Verification items for the finished model (mm, model axes). Face numbers are marked on the shaded views. Coordinates: 2 decimals unless noted, no trailing zeros. Loops run counter-clockwise (first coordinate to the right, second up) from the corner with the lowest first, then second, coordinate; pieces in that order, holes last. Notation, with made-up numbers: (9.5, 70) -> (53.5, 70) arc R12 ccw to (53.5, 89) -> close; hole circle Ø8 at (16, 40). An arc over 180 degrees is marked (long way). Write item = value, one per line.
```python
from build123d import *

# Parameters (mm, degrees)
SKETCH1_R           = 45
SKETCH1_R_2         = 2
SKETCH1_R_3         = 20
BOSS_EXTRUDE1_DEPTH = 5
BOSS_EXTRUDE2_START = 5
SKETCH2_R           = 45
SKETCH2_R_2         = 20
BOSS_EXTRUDE2_DEPTH = 5
SKETCH3_R           = 45
BOSS_EXTRUDE3_DEPTH = 20
CUT_EXTRUDE1_START  = -20
SKETCH4_R           = 2
CUT_EXTRUDE1_DEPTH  = 20


with BuildPart() as part:
    # Sketch1 → Boss-Extrude1 (new body)
    with BuildSketch(Plane(origin=(0, 0, 0), x_dir=(1, 0, 0), z_dir=(0, 1, 0))):
        with Locations(Location((0, 0, 0), (0, 0, 270))):
            Circle(SKETCH1_R)
        with Locations(Location((0, 39, 0), (0, 0, 270))):
            Circle(SKETCH1_R_2, mode=Mode.SUBTRACT)
        with Locations(Location((13.33878559, 36.648012211, 0), (0, 0, 270))):
            Circle(SKETCH1_R_2, mode=Mode.SUBTRACT)
        with Locations(Location((25.068716778, 29.875733282, 0), (0, 0, 270))):
            Circle(SKETCH1_R_2, mode=Mode.SUBTRACT)
        with Locations(Location((33.774990748, 19.5, 0), (0, 0, 270))):
            Circle(SKETCH1_R_2, mode=Mode.SUBTRACT)
        with Locations(Location((38.407502367, 6.772278929, 0), (0, 0, 270))):
            Circle(SKETCH1_R_2, mode=Mode.SUBTRACT)
        with Locations(Location((38.407502367, -6.772278929, 0), (0, 0, 270))):
            Circle(SKETCH1_R_2, mode=Mode.SUBTRACT)
        with Locations(Location((33.774990748, -19.5, 0), (0, 0, 270))):
            Circle(SKETCH1_R_2, mode=Mode.SUBTRACT)
        with Locations(Location((25.068716778, -29.875733282, 0), (0, 0, 270))):
            Circle(SKETCH1_R_2, mode=Mode.SUBTRACT)
        with Locations(Location((13.33878559, -36.648012211, 0), (0, 0, 270))):
            Circle(SKETCH1_R_2, mode=Mode.SUBTRACT)
        with Locations(Location((0, -39, 0), (0, 0, 270))):
            Circle(SKETCH1_R_2, mode=Mode.SUBTRACT)
        with Locations(Location((-13.33878559, -36.648012211, 0), (0, 0, 270))):
            Circle(SKETCH1_R_2, mode=Mode.SUBTRACT)
        with Locations(Location((-25.068716778, -29.875733282, 0), (0, 0, 270))):
            Circle(SKETCH1_R_2, mode=Mode.SUBTRACT)
        with Locations(Location((-33.774990748, -19.5, 0), (0, 0, 270))):
            Circle(SKETCH1_R_2, mode=Mode.SUBTRACT)
        with Locations(Location((-38.407502367, -6.772278929, 0), (0, 0, 270))):
            Circle(SKETCH1_R_2, mode=Mode.SUBTRACT)
        with Locations(Location((-38.407502367, 6.772278929, 0), (0, 0, 270))):
            Circle(SKETCH1_R_2, mode=Mode.SUBTRACT)
        with Locations(Location((-33.774990748, 19.5, 0), (0, 0, 270))):
            Circle(SKETCH1_R_2, mode=Mode.SUBTRACT)
        with Locations(Location((-25.068716778, 29.875733282, 0), (0, 0, 270))):
            Circle(SKETCH1_R_2, mode=Mode.SUBTRACT)
        with Locations(Location((-13.33878559, 36.648012211, 0), (0, 0, 270))):
            Circle(SKETCH1_R_2, mode=Mode.SUBTRACT)
        with Locations(Location((0, 0, 0), (0, 0, 270))):
            Circle(SKETCH1_R_3, mode=Mode.SUBTRACT)
    extrude(amount=BOSS_EXTRUDE1_DEPTH)

    # Sketch2 → Boss-Extrude2 (add)
    with BuildSketch(Plane.XZ.offset(BOSS_EXTRUDE2_START)):
        with Locations(Location((0, 0, 0), (0, 0, 270))):
            Circle(SKETCH2_R)
        with Locations(Location((0, 0, 0), (0, 0, 270))):
            Circle(SKETCH2_R_2, mode=Mode.SUBTRACT)
    extrude(amount=-BOSS_EXTRUDE2_DEPTH)

    # Sketch3 → Boss-Extrude3 (add)
    with BuildSketch(Plane(origin=(0, 0, 0), x_dir=(1, 0, 0), z_dir=(0, 1, 0))):
        with Locations(Location((0, 0, 0), (0, 0, 90))):
            Circle(SKETCH3_R)
        with BuildLine():
            ThreePointArc((-33.939016056, 17.506737424), (-32.04293994, 18.5), (-32.130787374, 20.638681372))
            ThreePointArc((-32.130787374, 20.638681372), (-31.849324915, 26.724756789), (-25.904586102, 28.058779107))
            ThreePointArc((-25.904586102, 28.058779107), (-23.783141558, 28.343644395), (-23.134219035, 30.383393091))
            ThreePointArc((-23.134219035, 30.383393091), (-20.788170452, 36.006167419), (-14.745680753, 35.226517926))
            ThreePointArc((-14.745680753, 35.226517926), (-12.654745303, 34.768626969), (-11.347322455, 36.463419192))
            ThreePointArc((-11.347322455, 36.463419192), (-7.219655832, 40.944702864), (-1.808228682, 38.145418796))
            ThreePointArc((-1.808228682, 38.145418796), (0, 37), (1.808228682, 38.145418796))
            ThreePointArc((1.808228682, 38.145418796), (7.219655832, 40.944702864), (11.347322455, 36.463419192))
            ThreePointArc((11.347322455, 36.463419192), (12.654745303, 34.768626969), (14.745680753, 35.226517926))
            ThreePointArc((14.745680753, 35.226517926), (20.788170452, 36.006167419), (23.134219035, 30.383393091))
            ThreePointArc((23.134219035, 30.383393091), (23.783141558, 28.343644395), (25.904586102, 28.058779107))
            ThreePointArc((25.904586102, 28.058779107), (31.849324915, 26.724756789), (32.130787374, 20.638681372))
            ThreePointArc((32.130787374, 20.638681372), (32.04293994, 18.5), (33.939016056, 17.506737424))
            ThreePointArc((33.939016056, 17.506737424), (39.068980747, 14.219946075), (37.251908557, 8.404640085))
            ThreePointArc((37.251908557, 8.404640085), (36.437886861, 6.424982574), (37.879899788, 4.843124835))
            ThreePointArc((37.879899788, 4.843124835), (41.576340904, 0), (37.879899788, -4.843124835))
            ThreePointArc((37.879899788, -4.843124835), (36.437886861, -6.424982574), (37.251908557, -8.404640085))
            ThreePointArc((37.251908557, -8.404640085), (39.068980747, -14.219946075), (33.939016056, -17.506737424))
            ThreePointArc((33.939016056, -17.506737424), (32.04293994, -18.5), (32.130787374, -20.638681372))
            ThreePointArc((32.130787374, -20.638681372), (31.849324915, -26.724756789), (25.904586102, -28.058779107))
            ThreePointArc((25.904586102, -28.058779107), (23.783141558, -28.343644395), (23.134219035, -30.383393091))
            ThreePointArc((23.134219035, -30.383393091), (20.788170452, -36.006167419), (14.745680753, -35.226517926))
            ThreePointArc((14.745680753, -35.226517926), (12.654745303, -34.768626969), (11.347322455, -36.463419192))
            ThreePointArc((11.347322455, -36.463419192), (7.219655832, -40.944702864), (1.808228682, -38.145418796))
            ThreePointArc((1.808228682, -38.145418796), (0, -37), (-1.808228682, -38.145418796))
            ThreePointArc((-1.808228682, -38.145418796), (-7.219655832, -40.944702864), (-11.347322455, -36.463419192))
            ThreePointArc((-11.347322455, -36.463419192), (-12.654745303, -34.768626969), (-14.745680753, -35.226517926))
            ThreePointArc((-14.745680753, -35.226517926), (-20.788170452, -36.006167419), (-23.134219035, -30.383393091))
            ThreePointArc((-23.134219035, -30.383393091), (-23.783141558, -28.343644395), (-25.904586102, -28.058779107))
            ThreePointArc((-25.904586102, -28.058779107), (-31.849324915, -26.724756789), (-32.130787374, -20.638681372))
            ThreePointArc((-32.130787374, -20.638681372), (-32.04293994, -18.5), (-33.939016056, -17.506737424))
            ThreePointArc((-33.939016056, -17.506737424), (-39.068980747, -14.219946075), (-37.251908557, -8.404640085))
            ThreePointArc((-37.251908557, -8.404640085), (-36.437886861, -6.424982574), (-37.879899788, -4.843124835))
            ThreePointArc((-37.879899788, -4.843124835), (-41.576340904, 0), (-37.879899788, 4.843124835))
            ThreePointArc((-37.879899788, 4.843124835), (-36.437886861, 6.424982574), (-37.251908557, 8.404640085))
            ThreePointArc((-37.251908557, 8.404640085), (-39.068980747, 14.219946075), (-33.939016056, 17.506737424))
        make_face(mode=Mode.SUBTRACT)
    extrude(amount=BOSS_EXTRUDE3_DEPTH)

    # Sketch4 → Cut-Extrude1 (cut)
    with BuildSketch(Plane(origin=(0, 20, 0), x_dir=(1, 0, 0), z_dir=(0, 1, 0)).offset(CUT_EXTRUDE1_START)):
        with Locations(Location((0, 39, 0), (0, 0, 270))):
            Circle(SKETCH4_R)
        with Locations(Location((13.33878559, 36.648012211, 0), (0, 0, 270))):
            Circle(SKETCH4_R)
        with Locations(Location((25.068716778, 29.875733282, 0), (0, 0, 270))):
            Circle(SKETCH4_R)
        with Locations(Location((33.774990748, 19.5, 0), (0, 0, 270))):
            Circle(SKETCH4_R)
        with Locations(Location((38.407502367, 6.772278929, 0), (0, 0, 270))):
            Circle(SKETCH4_R)
        with Locations(Location((38.407502367, -6.772278929, 0), (0, 0, 270))):
            Circle(SKETCH4_R)
        with Locations(Location((33.774990748, -19.5, 0), (0, 0, 270))):
            Circle(SKETCH4_R)
        with Locations(Location((25.068716778, -29.875733282, 0), (0, 0, 270))):
            Circle(SKETCH4_R)
        with Locations(Location((13.33878559, -36.648012211, 0), (0, 0, 270))):
            Circle(SKETCH4_R)
        with Locations(Location((0, -39, 0), (0, 0, 270))):
            Circle(SKETCH4_R)
        with Locations(Location((-13.33878559, -36.648012211, 0), (0, 0, 270))):
            Circle(SKETCH4_R)
        with Locations(Location((-25.068716778, -29.875733282, 0), (0, 0, 270))):
            Circle(SKETCH4_R)
        with Locations(Location((-33.774990748, -19.5, 0), (0, 0, 270))):
            Circle(SKETCH4_R)
        with Locations(Location((-38.407502367, -6.772278929, 0), (0, 0, 270))):
            Circle(SKETCH4_R)
        with Locations(Location((-38.407502367, 6.772278929, 0), (0, 0, 270))):
            Circle(SKETCH4_R)
        with Locations(Location((-33.774990748, 19.5, 0), (0, 0, 270))):
            Circle(SKETCH4_R)
        with Locations(Location((-25.068716778, 29.875733282, 0), (0, 0, 270))):
            Circle(SKETCH4_R)
        with Locations(Location((-13.33878559, 36.648012211, 0), (0, 0, 270))):
            Circle(SKETCH4_R)
    extrude(amount=CUT_EXTRUDE1_DEPTH, mode=Mode.SUBTRACT)


solid = part.part
```
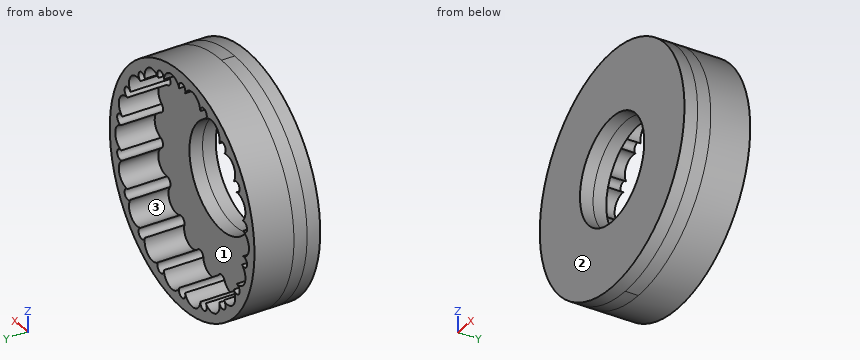
1) Sectioned sample at D-D, the plane x = -30. Record the cut outline in (y, z), plus the area to 3 significant figures.
Ans:
outline = (-5, -33.54) -> (20, -33.54) -> (20, -28.1) -> (5, -28.1) -> (5, 28.1) -> (20, 28.1) -> (20, 33.54) -> (-5, 33.54) -> close
area = 834 mm2
2) Sectioned sample at C-C, the plane y = 1.5. Count the separate pieces of the cut face and the enclosed holes in it, plus the area to 3 significant figures.
Ans:
separate_pieces = 1
enclosed_holes = 19
area = 4,880 mm2
3) Release check for a two-part mould opening along Z. For the marked faces 1, 2 and 3 record: pulls with the +Z half, pulls with the -Z half, needs draft (parallel to the pull), parting line crosses it, or undercut.
Ans:
face_1 = undercut
face_2 = needs draft
face_3 = undercut
4) Depth check by flat-ended pin: pin 1 Ø1.5 at (x, z) = (25, 4) entering from +Y; pin 2 Ø2 at (x, z) = (-25.5, 30) entering from +Y; pin 3 Ø1 at (y, z) = (4.5, 1) entering from -X. Enter the tip coordinate at first touch or a pass-through.
Ans:
pin_1 = 5
pin_2 = 0
pin_3 = -45
5) Sectioned sample at B-B, the plane x = 10. Record the cut outline in (y, z), plus the area to 3 significant figures.
Ans:
outline = (-5, -43.87) -> (20, -43.87) -> (20, -39.45) -> (5, -39.45) -> (5, -17.32) -> (-5, -17.32) -> close; (-5, 17.32) -> (5, 17.32) -> (5, 39.45) -> (20, 39.45) -> (20, 43.87) -> (-5, 43.87) -> close
area = 664 mm2
6) Sectioned sample at A-A, the plane z = 0. Record the cut outline in (x, y), plus the area to 3 significant figures.
Ans:
outline = (-45, -5) -> (-20, -5) -> (-20, 5) -> (-41.58, 5) -> (-41.58, 20) -> (-45, 20) -> close; (20, -5) -> (45, -5) -> (45, 20) -> (41.58, 20) -> (41.58, 5) -> (20, 5) -> close
area = 603 mm2
7) Material ranges on line 1 (Z direction, x = -33, y = 1.5); line 2 (Y direction, x = 8.5, z = -28.5); line 3 (Z direction, x = 35, y = 18.5), recorded low to high.
Ans:
line_1 = -30.59 to -21.34, -17.66 to 17.66, 21.34 to 30.59
line_2 = -5 to 5
line_3 = -28.28 to -21.08, -17.92 to -17.48, 17.48 to 17.92, 21.08 to 28.28
